Check sheet for the modelled part. Datum: model origin and axes. Units: mm. A direction names the side the tool comes from. Round coordinates to 2 decimals unless told otherwise and drop trailing zeros. Order: outer loops, then holes, each group sorted by start corner. A loop starts at its lowest first (then second) coordinate and runs counter-clockwise, first axis right, second up. Notation, with made-up numbers: (-38, 88) -> (19, 88) arc R25 ccw to (19, 119) -> close; hole circle Ø9 at (4, 2). An arc over 180 degrees is marked (long way). Answer in a Markdown table with one row per item. Add a question column.
1. Sectioned sample at C-C, the plane y = 0. Record the boundary of the cut face in (x, z), then the cut area to 3 significant figures.
2. Sectioned sample at A-A, the plane z = 1.7. Record the boundary of the cut face in (x, y).
3. Sectioned sample at D-D, the plane x = 21. Record the boundary of the cut face in (y, z).
4. Depth check by flat-ended pin: P1, Ø1.9, axis at x = -25.5, z = 2.5, coming from the +Y side. Enter the tip coordinate at first touch or a pass-through.
5. Draft check along X on faces 3 (the flat face through (-22, -1.95, 2)), 4 (the cylindrical face through (-0.38, -41.75, 1.87)), 5 (the cylindrical face through (0.15, 7.45, 1.87)), 6 (the cylindrical face through (1.437, -1.318, 1.873)). Enter one of: +X half, -X half, draft (parallel to the pull), parting line (faces both ways), or undercut.
6. Sectioned sample at B-B, the plane x = 0. Record the boundary of the cut face in (y, z).
7. Access from +Z, -Z, +X, -X, +Y, -Y to the whole of each face (thin tool, end or side, straight path). Record for faces 1 (the flat face through (23, -1.95, 2)), 2 (the flat face through (-30, -44.15, 2)).
8. Material ranges on L1, parallel to Y at x = 0, z = 2.4; L2, parallel to Y at x = 9.5, z = 0.8; L3, parallel to X at y = 5, z = 3.55, recorded low to high. Write a range as from..to.
```python
from build123d import *

# Parameters (mm, degrees)
SKETCH1_R      = 1.95
EXTRUDE1_DEPTH = 3.8


with BuildPart() as part:
    # Sketch1 → Extrude1 (new body)
    with BuildSketch(Plane.XY):
        with BuildLine():
            Line((26.8, -44.15), (33.8, -44.15))
            ThreePointArc((33.8, -44.15), (34.507106781, -43.857106781), (34.8, -43.15))
            Line((34.8, -43.15), (34.8, -2.95))
            ThreePointArc((34.8, -2.95), (34.507106781, -2.242893219), (33.8, -1.95))
            Line((33.8, -1.95), (11.054410884, -1.95))
            ThreePointArc((11.054410884, -1.95), (8.625166624, -1.056794064), (7.35315724, 1.197321429))
            ThreePointArc((7.35315724, 1.197321429), (0, 7.45), (-7.35315724, 1.197321429))
            ThreePointArc((-7.35315724, 1.197321429), (-8.625166624, -1.056794064), (-11.054410884, -1.95))
            Line((-11.054410884, -1.95), (-33.8, -1.95))
            ThreePointArc((-33.8, -1.95), (-34.507106781, -2.242893219), (-34.8, -2.95))
            Line((-34.8, -2.95), (-34.8, -43.15))
            ThreePointArc((-34.8, -43.15), (-34.507106781, -43.857106781), (-33.8, -44.15))
            Line((-33.8, -44.15), (-26.8, -44.15))
            ThreePointArc((-26.8, -44.15), (0, -41.75), (26.8, -44.15))
        make_face()
        with Locations(Location((0, 0, 0), (0, 0, 180))):
            Circle(SKETCH1_R, mode=Mode.SUBTRACT)
    extrude(amount=EXTRUDE1_DEPTH)


solid = part.part
```
Answer key:
| question | item | result |
|---|---|---|
| 1 | outline | (-7.76, 0) -> (-1.95, 0) -> (-1.95, 3.8) -> (-7.76, 3.8) -> close; (1.95, 0) -> (7.76, 0) -> (7.76, 3.8) -> (1.95, 3.8) -> close |
| 1 | area | 44.2 mm² |
| 2 | outline | (-34.8, -43.15) arc R1 ccw to (-33.8, -44.15) -> (-26.8, -44.15) arc R150.83 cw to (26.8, -44.15) -> (33.8, -44.15) arc R1 ccw to (34.8, -43.15) -> (34.8, -2.95) arc R1 ccw to (33.8, -1.95) -> (11.05, -1.95) arc R3.75 cw to (7.35, 1.2) arc R7.45 ccw to (-7.35, 1.2) arc R3.75 cw to (-11.05, -1.95) -> (-33.8, -1.95) arc R1 ccw to (-34.8, -2.95) -> close; hole circle Ø3.9 at (0, 0) |
| 3 | outline | (-43.22, 0) -> (-1.95, 0) -> (-1.95, 3.8) -> (-43.22, 3.8) -> close |
| 4 | P1 | stops at y = -1.95 |
| 5 | face 3 | draft |
| 5 | face 4 | undercut |
| 5 | face 5 | parting line |
| 5 | face 6 | undercut |
| 6 | outline | (-41.75, 0) -> (-1.95, 0) -> (-1.95, 3.8) -> (-41.75, 3.8) -> close; (1.95, 0) -> (7.45, 0) -> (7.45, 3.8) -> (1.95, 3.8) -> close |
| 7 | face 1 | +Z, -Z, +X, +Y |
| 7 | face 2 | +Z, -Z, +X, -X, -Y |
| 8 | L1 | y = -41.75..-1.95, 1.95..7.45 |
| 8 | L2 | y = -42.05..-1.61 |
| 8 | L3 | x = -5.52..5.52 |
